Build history of the part. All positions in model axes, mm. Face numbers are marked on the shaded views. A direction names the side the tool comes from. Give positions to 0.01 mm unless a question says otherwise; leave off trailing zeros. Write each loop counter-clockwise with the first axis right and the second up, starting at its lowest first coordinate (ties: lowest second). Pieces come first, ordered by that corner, then holes. Notation, with made-up numbers: M 81,36.5 L 91,36.5 A21 ccw 91,60.5 Z; hole C 74.25,16 d6. An arc over 180 degrees is marked long. Return JSON: item names as keys, results as strings. Group by question number.
Q1. Band-saw the part on A-A, the plane y = 0. Give the cut face in (x, z), then the cut area to 3 significant figures.
Q2. Tool access for the marked faces 1 and 2: list every direction of +Z, -Z, +X, -X, +Y, -Y with a clear straight run to the whole face (end or side of a thin tool).
Q3. Wall check: probe 1 along X at (y, z) = (20, 3.05); probe 2 along Z at (x, y) = (-11, 38.5); probe 3 along X at (y, z) = (22, 3). Give the ranges that are in metal, low to high.
Q4. Flat gauge pins, fed straight in: pin 1 Ø4.5 at (x, z) = (-37.5, 7) entering from -Y; pin 2 Ø3 at (x, z) = (-40.5, 9) entering from +Y; pin 3 Ø4 at (x, y) = (15.5, 34.5) entering from +Z. Where does each tip first touch, or does it go through?
Q5. Band-saw the part on B-B, the plane x = 0. Give the cut face in (y, z), then the cut area to 3 significant figures.
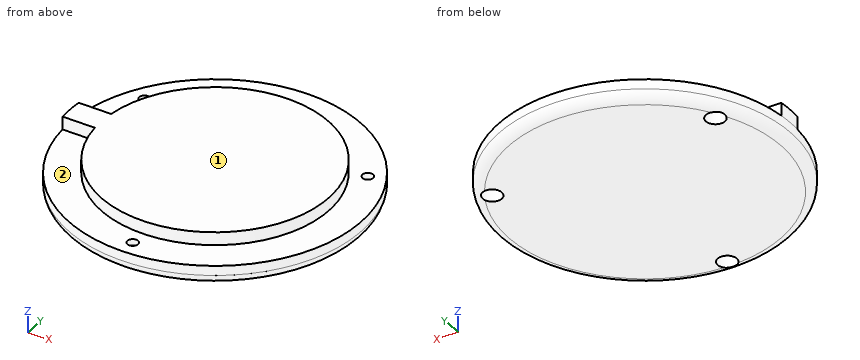
from build123d import *

# Parameters (mm, degrees)
ESBO_O1_R                = 45
RESSALTO_EXTRUS_O1_DEPTH = 6
RESSALTO_EXTRUS_O2_DEPTH = 4
ESBO_O4_R                = 1.65
CORTE_EXTRUS_O1_DEPTH    = 2
ESBO_O5_R                = 2.95
CORTE_EXTRUS_O2_DEPTH    = 4
FILETE1_R                = 3


with BuildPart() as part:
    # Esboço1 → Ressalto-extrusão1 (new body)
    with BuildSketch(Plane.XY):
        Circle(ESBO_O1_R)
    extrude(amount=RESSALTO_EXTRUS_O1_DEPTH)

    # Esboço3 → Ressalto-extrusão2 (add)
    with BuildSketch(Plane.XY.offset(6)):
        with BuildLine():
            Line((-34.776392855, 3.95), (-44.826303662, 3.95))
            ThreePointArc((-44.826303662, 3.95), (-45, 0), (-44.826303662, -3.95))
            Line((-44.826303662, -3.95), (-34.776392855, -3.95))
            ThreePointArc((-34.776392855, -3.95), (35, 0), (-34.776392855, 3.95))
        make_face()
    extrude(amount=RESSALTO_EXTRUS_O2_DEPTH)

    # Esboço4 → Corte-extrusão1 (cut)
    with BuildSketch(Plane.XY.offset(6)):
        with Locations((0, -40)):
            Circle(ESBO_O4_R)
        with Locations((-34.641016151, 20)):
            Circle(ESBO_O4_R)
        with Locations((34.641016151, 20)):
            Circle(ESBO_O4_R)
    extrude(amount=-CORTE_EXTRUS_O1_DEPTH, mode=Mode.SUBTRACT)

    # Esboço5 → Corte-extrusão2 (cut)
    with BuildSketch(Plane.XY.offset(4)):
        with Locations((0, -40)):
            Circle(ESBO_O5_R)
        with Locations((-34.641016151, 20)):
            Circle(ESBO_O5_R)
        with Locations((34.641016151, 20)):
            Circle(ESBO_O5_R)
    extrude(amount=-CORTE_EXTRUS_O2_DEPTH, mode=Mode.SUBTRACT)

    # Filete1
    # the kernel refuses this fillet: 3 mm, written as the material it takes off along each edge
    with BuildSketch(Plane(origin=(0, 0, 0), x_dir=(1, 0, 0), z_dir=(0, -1, 0))) as filete1_piece_1:
        with BuildLine():
            CenterArc((45 - FILETE1_R, FILETE1_R), FILETE1_R, 270, 90)
            Line((45 - FILETE1_R, 0), (45, 0))
            Line((45, 0), (45, FILETE1_R))
        make_face()
    revolve(axis=Axis((0, 0, 0), (0, 0, 1)), mode=Mode.SUBTRACT)


solid = part.part
From the geometry:
{
 "1": {"outline": "M -45,3 A3 ccw -42,0 L 42,0 A3 ccw 45,3 L 45,6 L 35,6 L 35,10 L -45,10 Z", "area": "856 mm^2"},
 "2": {"face 1": "+Z, +X, -X, +Y, -Y", "face 2": "+Z"},
 "3": {"probe 1": "x = -40.31 to -37.59, -31.69 to 31.69, 37.59 to 40.31", "probe 2": "z = 0 to 6", "probe 3": "x = -39.26 to -36.81, -32.47 to 32.47, 36.81 to 39.26"},
 "4": {"pin 1": "stops at y = -27.67", "pin 2": "stops at y = 3.95", "pin 3": "stops at z = 6"},
 "5": {"outline": "M -45,3 A3 ccw -42.95,0.15 L -42.95,4 L -41.65,4 L -41.65,6 L -45,6 Z; M -38.35,4 L -37.05,4 L -37.05,0 L 42,0 A3 ccw 45,3 L 45,6 L 35,6 L 35,10 L -35,10 L -35,6 L -38.35,6 Z", "area": "786 mm^2"}
}
